```python
from build123d import *

# Parameters (mm, degrees)
F0_W     = 254
F0_H     = 304.8
F1_DEPTH = 63.5
F2_SIZE  = 5.08


with BuildPart() as f1:
    # F0 (on Top) → F1 (new body)
    with BuildSketch(Plane.XY):
        Rectangle(F0_W, F0_H)
        with BuildLine():
            ThreePointArc((-114.3, 114.3), (-106.860512, 132.260512), (-88.9, 139.7))
            Line((-88.9, 139.7), (88.9, 139.7))
            ThreePointArc((88.9, 139.7), (106.860512, 132.260512), (114.3, 114.3))
            Line((114.3, 114.3), (114.3, -114.3))
            ThreePointArc((114.3, -114.3), (106.860512, -132.260512), (88.9, -139.7))
            Line((88.9, -139.7), (-88.9, -139.7))
            ThreePointArc((-88.9, -139.7), (-106.860512, -132.260512), (-114.3, -114.3))
            Line((-114.3, -114.3), (-114.3, 114.3))
        make_face(mode=Mode.SUBTRACT)
    extrude(amount=F1_DEPTH)

    # F2
    f2_edges = [f1.edges().sort_by_distance(p)[0] for p in [
        (-127, 152.4, 31.75),
        (127, 152.4, 31.75),
        (127, -152.4, 31.75),
        (-127, -152.4, 31.75),
    ]]
    chamfer(f2_edges, length=F2_SIZE)


solid = f1.part
```
Check sheet for the modelled part. Datum: model origin and axes. Units: mm. A direction names the side the tool comes from. Give positions to 0.01 mm unless a question says otherwise; leave off trailing zeros. Loops run counter-clockwise (first coordinate to the right, second up) from the corner with the lowest first, then second, coordinate; pieces in that order, holes last. Notation, with made-up numbers: (48.25, 34) - (104.25, 34) arc R10 ccw to (104.25, 47) - close; hole circle Ø7 at (13.25, 31.25). An arc over 180 degrees is marked (long way). One line per question, with ' | ' between items. Start each with the question number.
1. Set-up check for faces 4 (the flat face through (-2, -152.4, 31)), 5 (the flat face through (1, -139.7, 31)): record each of +Z, -Z, +X, -X, +Y, -Y from which the full face is reachable in a straight line by a thin tool's end or side.
2. Cross-section at A-A, the plane z = 55.5. Enter the section's corners in (x, y), plus the area to 3 significant figures.
3. Cross-section at C-C, the plane x = 40. Enter the section's corners in (y, z), plus the area to 3 significant figures.
4. Draft check along Y on faces 1 (the flat face through (127, -2, 31)), 2 (the cylindrical face through (-106.66, -132.46, 31.31)), 3 (the flat face through (-2, 152.4, 31)). Enter one of: released by +Y, released by -Y, zero draft, split by the parting line, or undercut.
5. Cross-section at B-B, the plane y = -85. Enter the section's corners in (x, z), plus the area to 3 significant figures.
6. Material ranges on line 1 along Y through (x, z) = (-47, 5.5); line 2 along X through (y, z) = (-76, 59); line 3 along Y through (x, z) = (-92.5, 19.5), recorded low to high. Write a range as [from, to].
Check result:
1) face 4: +Z, -Z, +X, -X, -Y | face 5: +Z, -Z
2) outline: (-127, -147.32) - (-121.92, -152.4) - (121.92, -152.4) - (127, -147.32) - (127, 147.32) - (121.92, 152.4) - (-121.92, 152.4) - (-127, 147.32) - close; hole (-114.3, -114.3) arc R25.4 ccw to (-88.9, -139.7) - (88.9, -139.7) arc R25.4 ccw to (114.3, -114.3) - (114.3, 114.3) arc R25.4 ccw to (88.9, 139.7) - (-88.9, 139.7) arc R25.4 ccw to (-114.3, 114.3) - close | area: 14,100 mm2
3) outline: (-152.4, 0) - (-139.7, 0) - (-139.7, 63.5) - (-152.4, 63.5) - close; (139.7, 0) - (152.4, 0) - (152.4, 63.5) - (139.7, 63.5) - close | area: 1,610 mm2
4) face 1: zero draft | face 2: undercut | face 3: released by +Y
5) outline: (-127, 0) - (-114.3, 0) - (-114.3, 63.5) - (-127, 63.5) - close; (114.3, 0) - (127, 0) - (127, 63.5) - (114.3, 63.5) - close | area: 1,610 mm2
6) line 1: y = [-152.4, -139.7], [139.7, 152.4] | line 2: x = [-127, -114.3], [114.3, 127] | line 3: y = [-152.4, -139.44], [139.44, 152.4]
